```python
from build123d import *

# Parameters (mm, degrees)
SKETCH1_W               = 48.3
SKETCH1_H               = 44
SKETCH1_R               = 1.6
SKETCH1_R_2             = 2.5527
SKETCH1_R_3             = 2.740604045
BOSS_EXTRUDE1_DEPTH     = 6.35
F_1_4_20_TAPPED_HOLE1_D = 5.1054
FILLET1_R               = 10


with BuildPart() as part:
    # Sketch1 → Boss-Extrude1 (new body)
    with BuildSketch(Plane.XY):
        with Locations((24.15, -22)):
            Rectangle(SKETCH1_W, SKETCH1_H)
        with Locations((7.5, -37)):
            Circle(SKETCH1_R, mode=Mode.SUBTRACT)
        with Locations((22.5, -9.3)):
            Circle(SKETCH1_R_2, mode=Mode.SUBTRACT)
        with Locations((35.2, -22)):
            Circle(SKETCH1_R_2, mode=Mode.SUBTRACT)
        with Locations((9.8, -22)):
            Circle(SKETCH1_R_2, mode=Mode.SUBTRACT)
        with Locations((22.5, -34.7)):
            Circle(SKETCH1_R_2, mode=Mode.SUBTRACT)
        with Locations((37.5, -37)):
            Circle(SKETCH1_R, mode=Mode.SUBTRACT)
        with Locations((37.5, -7)):
            Circle(SKETCH1_R, mode=Mode.SUBTRACT)
        with Locations((7.5, -7)):
            Circle(SKETCH1_R, mode=Mode.SUBTRACT)
        with Locations((22.5, -22)):
            Circle(SKETCH1_R_3, mode=Mode.SUBTRACT)
    extrude(amount=BOSS_EXTRUDE1_DEPTH)

    # 1/4-20 Tapped Hole1 (through all)
    with Locations(Plane(origin=(22.5, -9.3, 6.35), x_dir=(1, 0, 0), z_dir=(0, 0, 1))):
        with Locations((0, 0), (12.7, -12.7), (-12.7, -12.7), (0, -25.4)):
            Hole(F_1_4_20_TAPPED_HOLE1_D / 2)

    # Fillet1
    fillet1_edges = [part.edges().sort_by_distance(p)[0] for p in [
        (0, 0, 3.175),
    ]]
    fillet(fillet1_edges, radius=FILLET1_R)


solid = part.part
```
Geometry check sheet. Reference: the model listing, model coordinates, mm. Round coordinates to 2 decimals unless told otherwise and drop trailing zeros. Order: outer loops, then holes, each group sorted by start corner. A loop starts at its lowest first (then second) coordinate and runs counter-clockwise, first axis right, second up. Notation, with made-up numbers: M 88,-17 L 114,-17 A30 ccw 114,19 Z; hole C -25.75,-35 d11. An arc over 180 degrees is marked long. Answer as CSV lines item,"result".
1) Sectioned sample at B-B on x = 22.5. Record the cut outline in (y, z), and give its area (3 significant figures).
Entries:
outline,"M -44,0 L -37.25,0 L -37.25,6.35 L -44,6.35 Z; M -32.15,0 L -24.74,0 L -24.74,6.35 L -32.15,6.35 Z; M -19.26,0 L -11.85,0 L -11.85,6.35 L -19.26,6.35 Z; M -6.75,0 L 0,0 L 0,6.35 L -6.75,6.35 Z"
area,"180 mm2"
2) Mould release check, pull along Y, two halves, no side actions. Record for faces 1 (the face through (29, -22, 0)), 2 (the face through (11.172, -19.848, 3.131)), 3 (the face through (24, -44, 3)): +Y half, -Y half, draft (parallel to the pull), parting line (faces both ways), or undercut.
Entries:
face 1,"draft"
face 2,"undercut"
face 3,"-Y half"
3) Sectioned sample at A-A on y = -22. Record the cut outline in (x, z).
Entries:
outline,"M 0,0 L 7.25,0 L 7.25,6.35 L 0,6.35 Z; M 12.35,0 L 19.76,0 L 19.76,6.35 L 12.35,6.35 Z; M 25.24,0 L 32.65,0 L 32.65,6.35 L 25.24,6.35 Z; M 37.75,0 L 48.3,0 L 48.3,6.35 L 37.75,6.35 Z"
4) Thickness scan on probe 1 along Y at (x, z) = (35.2, 2.75); probe 2 along X at (y, z) = (-34.7, 3.75); probe 3 along Y at (x, z) = (7.5, 2.75). Record the ranges inside material, lowest first. Write a range as [from, to].
Entries:
probe 1,"[-44, -24.55], [-19.45, 0]"
probe 2,"[0, 19.95], [25.05, 48.3]"
probe 3,"[-44, -38.6], [-35.4, -23.11], [-20.89, -8.6], [-5.4, -0.32]"
5) Gauge pin test, flat ends, axial feed: pin 1 Ø4 at (x, y) = (22.5, -9.3) entering from -Z; pin 2 Ø4 at (x, y) = (37.5, -37) entering from +Z. Record the tip position at first contact, or that the pin passes through.
Entries:
pin 1,"through"
pin 2,"z = 6.35"
6) Sectioned sample at C-C on z = 2.5. Give the number of separate pieces and of enclosed holes in the cut face, and give its area (3 significant figures).
Entries:
separate pieces,"1"
enclosed holes,"9"
area,"1,970 mm2"
